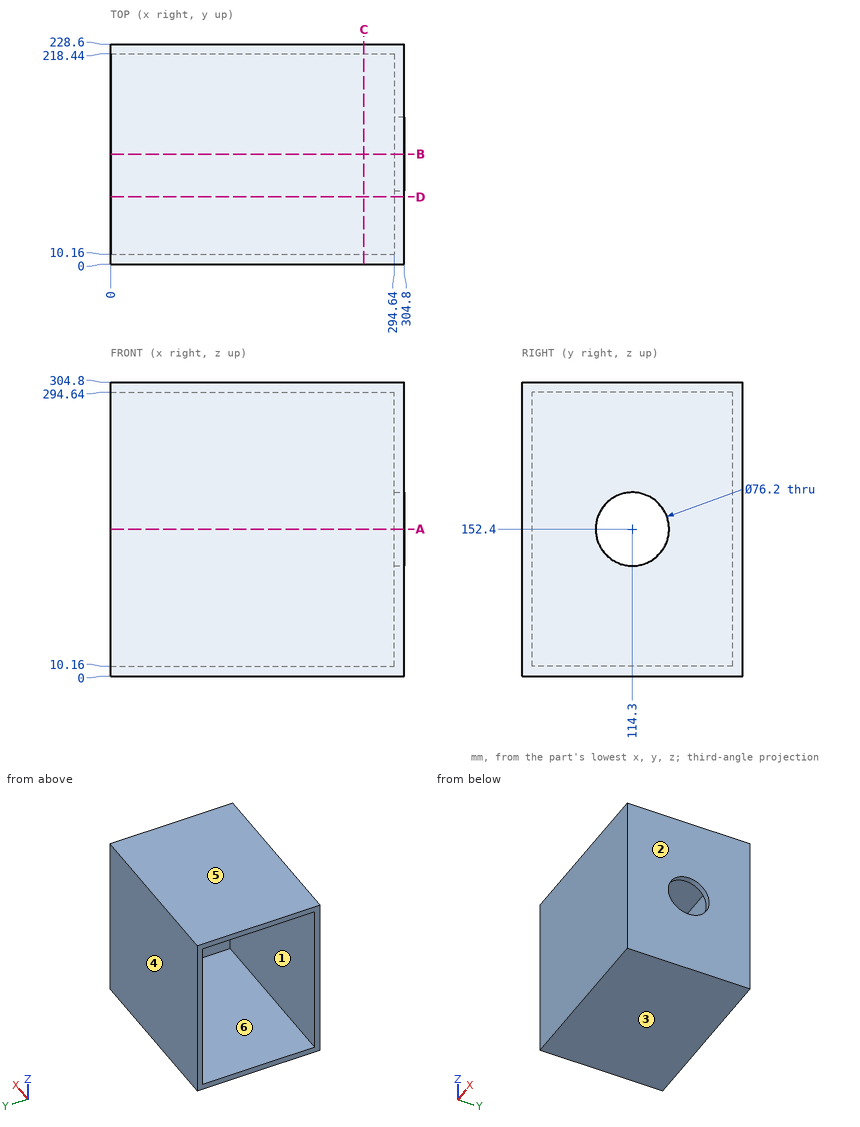
Can you work these out from the drawing? Everything is in mm from the part's minimum corner. A direction names the side the tool comes from. Round coordinates to 2 decimals unless told otherwise and drop trailing zeros. Write each loop counter-clockwise with the first axis right and the second up, starting at its lowest first coordinate (ties: lowest second). Pieces come first, ordered by that corner, then holes.
1. If we mould it in two halves opening along Z, with no side actions, what happens to the marked faces 3, 4, 5 and 6? For each: released by +Z, released by -Z, zero draft, split by the parting line, or undercut.
2. Suppose I cut it at A-A (z = 152.4). List the corners of the cut face in (x, y) for me.
3. For the marked faces 1 and 2, which set-ups out of +Z, -Z, +X, -X, +Y, -Y let a thin tool reach every point of the face, with its end or its side?
4. Will these pins go through, and if not, where does the flat tip stop? pin 1 Ø5 at (y, z) = (130, 182.5) entering from +X; pin 2 Ø1 at (y, z) = (167.5, 62.5) entering from -X.
5. Suppose I cut it at B-B (y = 114.3). List the corners of the cut face in (x, z) for me.
6. Suppose I cut it at C-C (x = 263). List the corners of the cut face in (y, z) for me, and give its area (3 significant figures).
7. I need wall thicknesses on L1, parallel to Z at x = 299, y = 114; L2, parallel to Z at x = 265.5, y = 88; L3, parallel to Y at x = 37.5, z = 269. Which ranges of each line are inside material? Lowest first, please.
8. Suppose I cut it at D-D (y = 70). List the corners of the cut face in (x, z) for me, and give its area (3 significant figures).
Answer sheet:
1. face 3: released by -Z
1. face 4: zero draft
1. face 5: released by +Z
1. face 6: undercut
2. outline: (0, 0) - (304.8, 0) - (304.8, 76.2) - (294.64, 76.2) - (294.64, 10.16) - (0, 10.16) - close; (0, 218.44) - (294.64, 218.44) - (294.64, 152.4) - (304.8, 152.4) - (304.8, 228.6) - (0, 228.6) - close
3. face 1: -X
3. face 2: +Z, -Z, +X, +Y, -Y
4. pin 1: passes through
4. pin 2: stops at x = 294.64
5. outline: (0, 0) - (304.8, 0) - (304.8, 114.3) - (294.64, 114.3) - (294.64, 10.16) - (0, 10.16) - close; (0, 294.64) - (294.64, 294.64) - (294.64, 190.5) - (304.8, 190.5) - (304.8, 304.8) - (0, 304.8) - close
6. outline: (0, 0) - (228.6, 0) - (228.6, 304.8) - (0, 304.8) - close; hole (10.16, 10.16) - (218.44, 10.16) - (218.44, 294.64) - (10.16, 294.64) - close
6. area: 10,400 mm2
7. L1: z = 0 to 114.3, 190.5 to 304.8
7. L2: z = 0 to 10.16, 294.64 to 304.8
7. L3: y = 0 to 10.16, 218.44 to 228.6
8. outline: (0, 0) - (304.8, 0) - (304.8, 304.8) - (0, 304.8) - (0, 294.64) - (294.64, 294.64) - (294.64, 10.16) - (0, 10.16) - close
8. area: 9,080 mm2
